For this review, use the dimensioned drawing (mm, ordinates from the lowest corner) and the shaded views. Give positions to 0.01 mm unless a question says otherwise; leave off trailing zeros. Order: outer loops, then holes, each group sorted by start corner. A loop starts at its lowest first (then second) coordinate and runs counter-clockwise, first axis right, second up. Notation, with made-up numbers: (84, -18.75) - (120, -18.75) arc R32 cw to (120, 10.25) - close; hole circle Ø11 at (30, -8.75). An arc over 180 degrees is marked (long way). One line per item, written item: value.
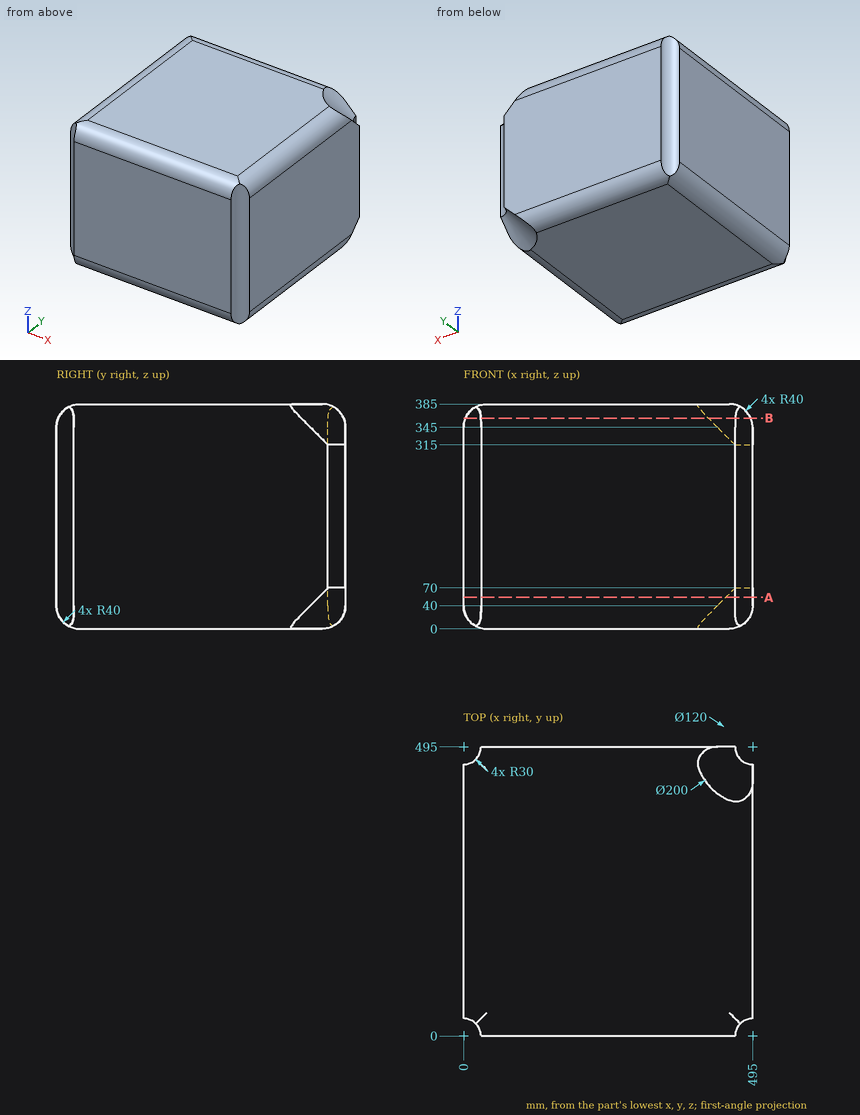
(1) Take a section at B-B (z = 361). Write out the cut boundary in (x, y).
Answers below:
outline: (3.34, 29.81) arc R30 cw to (29.81, 3.34) - (465.19, 3.34) arc R30 cw to (491.66, 29.81) - (491.66, 419.07) arc R76 cw to (419.07, 491.66) - (29.81, 491.66) arc R30 cw to (3.34, 465.19) - close
(2) Take a section at A-A (z = 54). Write out the cut boundary in (x, y), then the cut area to 3 significant figures.
Answers below:
outline: (0, 30) arc R30 cw to (30, 0) - (465, 0) arc R30 cw to (495, 30) - (495, 449) arc R46 cw to (449, 495) - (30, 495) arc R30 cw to (0, 465) - close
area: 241,000 mm^2
(3) Wall thickness on line 1 (X direction, y = 202.5, z = 346); line 2 (X direction, y = 45.5, z = 352); line 3 (Z direction, x = 203.5, y = 34.5): over which ranges is each line inside the solid? List them lowest first. Write a range as from..to.
Answers below:
line 1: x = 0.01..494.99
line 2: x = 0.62..494.38
line 3: z = 0.38..384.62
